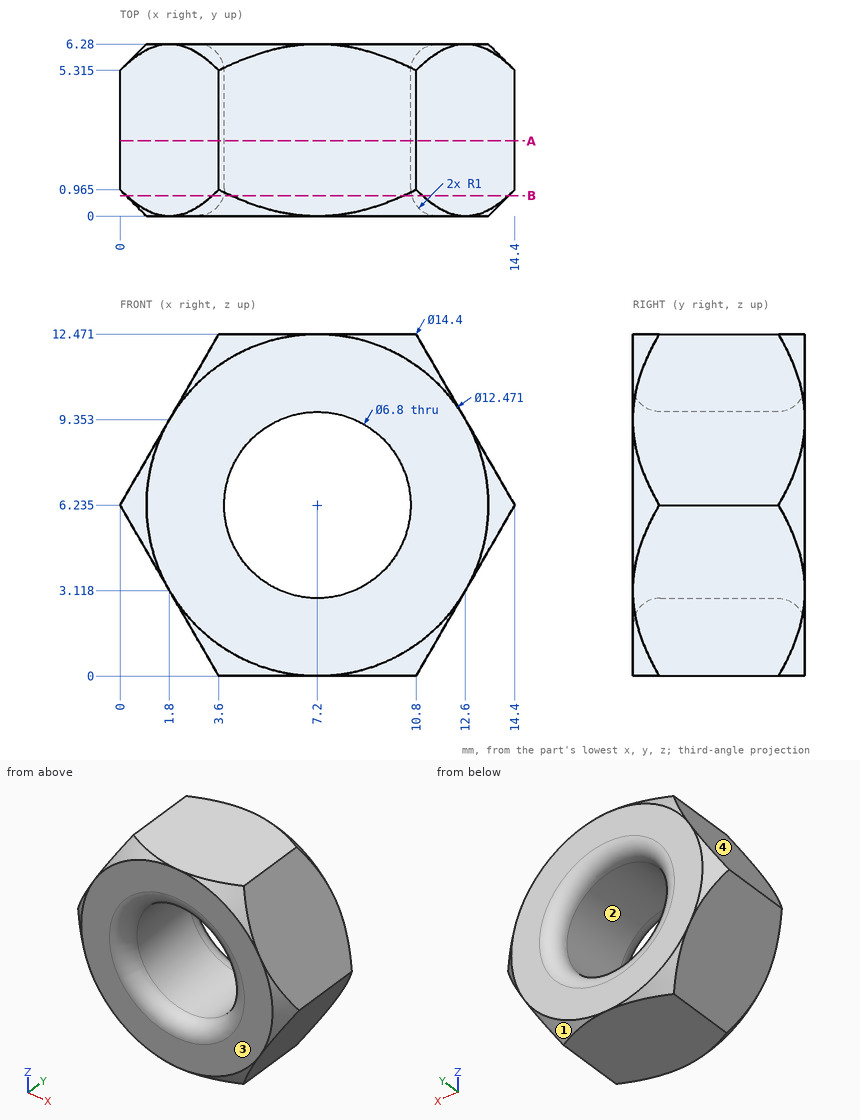
Input: dimensioned drawing with shaded views. Units: mm. Origin: part minimum x, y, z. Round coordinates to 2 decimals unless told otherwise and drop trailing zeros. Order: outer loops, then holes, each group sorted by start corner. A loop starts at its lowest first (then second) coordinate and runs counter-clockwise, first axis right, second up. Notation, with made-up numbers: M 5,66 L 64,66 A17 cw 64,94 Z; hole C 23,11 d5. An arc over 180 degrees is marked long. Use one line per item in the form item = value. Start each with the question number.
Q1. Pin query (flat end, axial travel): pin 1 Ø2 at (y, z) = (2, 11) entering from -X; pin 2 Ø3 at (y, z) = (3.5, 1.5) entering from +X; pin 3 Ø2 at (y, z) = (2.5, 2) entering from -X; pin 4 Ø5.5 at (x, z) = (7.2, 6.24) entering from +Y. Return the tip coordinate at first contact, or that it passes through.
Q2. Cut plane A-A (y = 2.75). Return loops of the section in (x, z) (1 decimal).
Q3. Mould query, pull axis X, two halves, no side actions, for the marked faces 1, 2, 3 and 4. Classes: +X half, -X half, draft (parallel to the pull), parting line (faces both ways), or undercut.
Q4. Cut plane B-B (y = 0.75). Return loops of the section in (x, z) (1 decimal).
Q5. Material intervals for line 1 (Y direction, x = 11.5, z = 6) (1 decimal); line 2 (Z direction, x = 7, y = 6) (1 decimal); line 3 (X direction, y = 1.5, z = 7.25) (1 decimal), sorted ascending. Write a range as [from, to].
Geometry results:
q1.pin_1 = 2.17
q1.pin_2 = 12.53
q1.pin_3 = 1.87
q1.pin_4 = through
q2.outline = M 0,6.2 L 3.6,0 L 10.8,0 L 14.4,6.2 L 10.8,12.5 L 3.6,12.5 Z; hole C 7.2,6.2 d6.8
q3.face_1 = +X half
q3.face_2 = undercut
q3.face_3 = draft
q3.face_4 = -X half
q4.outline = M 0.2,5.8 L 3.4,0.4 A7 ccw 4.1,0 L 10.3,0 A7 ccw 11,0.4 L 14.2,5.8 A7 ccw 14.2,6.6 L 11,12.1 A7 ccw 10.3,12.5 L 4.1,12.5 A7 ccw 3.4,12.1 L 0.2,6.6 A7 ccw Z; hole C 7.2,6.2 d6.9
q5.line_1 = [0, 6.3]
q5.line_2 = [0, 2.5], [9.9, 12.5]
q5.line_3 = [0.6, 4], [10.4, 13.8]
